The listing builds one solid part. Answer for the finished solid, in the listing's coordinates (mm). A direction names the side the tool comes from. Give positions to 0.01 mm unless a question says otherwise; leave off trailing zeros. Loops run counter-clockwise (first coordinate to the right, second up) from the corner with the lowest first, then second, coordinate; pieces in that order, holes last. Notation, with made-up numbers: M -37.5,51.25 L -14.5,51.25 A26 cw -14.5,71.25 Z; hole C -1.5,75.25 d10. An arc over 180 degrees is marked long. Use one line per item in the form item = value. Start each with the question number.
1. The part is cut by section D-D (y = -10). Write down the section's boundary in (x, z).
2. The part is cut by section C-C (z = 2.35). Give the number of separate pieces and of enclosed holes in the cut face, and give its area (3 significant figures).
3. The part is cut by section A-A (y = -26). Write down the section's boundary in (x, z).
4. The mould has two halves that part along X. Classify faces 4 (the face through (-19.81, 29.91, 1.48)), 5 (the face through (-44.2, -30, 1)), 6 (the face through (33, -32, 1)): released by +X, released by -X, zero draft, split by the parting line, or undercut.
5. The part is cut by section B-B (x = 20). Write down the section's boundary in (y, z).
6. Each of these flat-tipped pins is pushed along its axis until it touches: pin 1 Ø0.9 at (x, z) = (45.5, 1.5) entering from -Y; pin 2 Ø1.5 at (y, z) = (6.5, 1.5) entering from -X; pin 3 Ø1.5 at (y, z) = (8.5, 1.5) entering from +X. Where does it stop, or does it pass through?
7. For faces 1 (the face through (22.25, -15, 1)), 2 (the face through (-46, 12, 1)), 3 (the face through (-44.2, 27, 1)), determine the directions among +Z, -Z, +X, -X, +Y, -Y from which every point of the face is accessible in a straight line to the end or side of a thin tool.
8. Straight lines are drawn through the part: line 1 (X direction, y = -11.5, z = 0.75); line 2 (X direction, y = -19, z = 0.9); line 3 (Y direction, x = -20, z = 2.4). For each, find the intervals that lie inside material, in ascending order. Write a range as from..to.
from build123d import *

# Parameters (mm, degrees)
SKETCH1_W           = 94.4
SKETCH1_H           = 64
BOSS_EXTRUDE1_DEPTH = 3
SKETCH2_W           = 3
SKETCH2_H           = 10
CUT_EXTRUDE1_DEPTH  = 3
SKETCH3_W           = 4.5
SKETCH3_H           = 34
CUT_EXTRUDE2_DEPTH  = 10
SKETCH4_R           = 1.4224
CUT_EXTRUDE3_DEPTH  = 6


with BuildPart() as part:
    # Sketch1 → Boss-Extrude1 (new body)
    with BuildSketch(Plane.XY):
        Rectangle(SKETCH1_W, SKETCH1_H)
    extrude(amount=BOSS_EXTRUDE1_DEPTH)

    # Sketch2 → Cut-Extrude1 (cut)
    with BuildSketch(Plane(origin=(0, 0, 0), x_dir=(-1, 0, 0), z_dir=(0, 0, -1))):
        with Locations((-45.7, 7)):
            Rectangle(SKETCH2_W, SKETCH2_H)
        with Locations((-45.7, 27)):
            Rectangle(SKETCH2_W, SKETCH2_H)
        with Locations((-45.7, -13)):
            Rectangle(SKETCH2_W, SKETCH2_H)
        with Locations((-45.7, -33)):
            Rectangle(SKETCH2_W, SKETCH2_H)
        with Locations((45.7, -33)):
            Rectangle(SKETCH2_W, SKETCH2_H)
        with Locations((45.7, -13)):
            Rectangle(SKETCH2_W, SKETCH2_H)
        with Locations((45.7, 7)):
            Rectangle(SKETCH2_W, SKETCH2_H)
        with Locations((45.7, 27)):
            Rectangle(SKETCH2_W, SKETCH2_H)
    extrude(amount=-CUT_EXTRUDE1_DEPTH, mode=Mode.SUBTRACT)

    # Sketch3 → Cut-Extrude2 (cut)
    with BuildSketch(Plane(origin=(0, 0, 0), x_dir=(-1, 0, 0), z_dir=(0, 0, -1))):
        with Locations((-20, -15)):
            Rectangle(SKETCH3_W, SKETCH3_H)
        with Locations((20, -15)):
            Rectangle(SKETCH3_W, SKETCH3_H)
    extrude(amount=-CUT_EXTRUDE2_DEPTH, mode=Mode.SUBTRACT)

    # Sketch4 → Cut-Extrude3 (cut)
    with BuildSketch(Plane(origin=(0, 0, 0), x_dir=(-1, 0, 0), z_dir=(0, 0, -1))):
        with Locations((-20, 28.5)):
            Circle(SKETCH4_R)
        with Locations((20, 28.5)):
            Circle(SKETCH4_R)
    extrude(amount=-CUT_EXTRUDE3_DEPTH, mode=Mode.SUBTRACT)


solid = part.part
Derived:
q1.outline = M -44.2,0 L -22.25,0 L -22.25,3 L -44.2,3 Z; M -17.75,0 L 17.75,0 L 17.75,3 L -17.75,3 Z; M 22.25,0 L 44.2,0 L 44.2,3 L 22.25,3 Z
q2.separate_pieces = 1
q2.enclosed_holes = 2
q2.area = 5,520 mm2
q3.outline = M -47.2,0 L -22.25,0 L -22.25,3 L -47.2,3 Z; M -17.75,0 L 17.75,0 L 17.75,3 L -17.75,3 Z; M 22.25,0 L 47.2,0 L 47.2,3 L 22.25,3 Z
q4.face_4 = undercut
q4.face_5 = released by -X
q4.face_6 = zero draft
q5.outline = M 2,0 L 27.08,0 L 27.08,3 L 2,3 Z; M 29.92,0 L 32,0 L 32,3 L 29.92,3 Z
q6.pin_1 = -28
q6.pin_2 = -44.2
q6.pin_3 = 44.2
q7.face_1 = +Z, -Z, -Y
q7.face_2 = +Z, -Z, -X
q7.face_3 = +Z, -Z, -X, +Y
q8.line_1 = -44.2..-22.25, -17.75..17.75, 22.25..44.2
q8.line_2 = -47.2..-22.25, -17.75..17.75, 22.25..47.2
q8.line_3 = 2..27.08, 29.92..32
